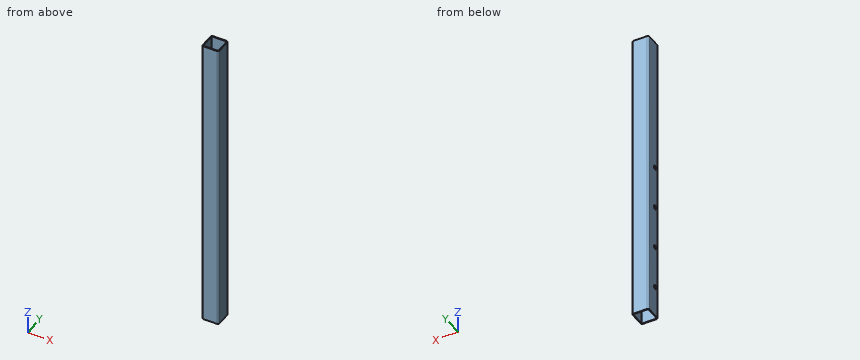
Autodesk Inventor part; units mm, degrees
ref_plane "Piano iniziale" through (0, 0, 0) normal (0, 0, 1) x (1, 0, 0)
ref_plane "Piano finale" through (0, 0, 720) normal (0, 0, 1) x (1, 0, 0)
ref_plane "YZ Plane" through (0, 0, 0) normal (1, 0, 0) x (0, 1, 0)
ref_plane "Piano iniziale" through (0, 0, 0) normal (0, 0, 1) x (1, 0, 0)
ref_plane "Piano finale" through (0, 0, 720) normal (0, 0, 1) x (1, 0, 0)
sketch "Schizzo" plane through (0, 0, 0) normal (0, 0, 1) x (1, 0, 0)
  line L0 (-20, -16) -> (-20, 16)
  line L1 (-16, 20) -> (16, 20)
  line L2 (20, 16) -> (20, -16)
  line L3 (16, -20) -> (-16, -20)
  arc A0 (-20, -16) -> (-16, -20) centre (-16, -16) ccw
  arc A1 (20, 16) -> (16, 20) centre (16, 16) ccw
  arc A2 (-16, 20) -> (-20, 16) centre (-16, 16) ccw
  arc A3 (16, -20) -> (20, -16) centre (16, -16) ccw
  arc A4 (-16, 18) -> (-18, 16) centre (-16, 16) ccw
  line L4 (-16, 18) -> (16, 18)
  arc A5 (18, 16) -> (16, 18) centre (16, 16) ccw
  line L5 (18, 16) -> (18, -16)
  arc A6 (16, -18) -> (18, -16) centre (16, -16) ccw
  line L6 (16, -18) -> (-16, -18)
  arc A7 (-18, -16) -> (-16, -18) centre (-16, -16) ccw
  line L7 (-18, -16) -> (-18, 16)
  line L8 (0, 29.1598) -> (0, -29.1598) construction
  line L9 (-29.1598, 0) -> (29.1598, 0) construction
  dimension "d7" = 4
  dimension "d9" = 40
  dimension "d11" = 40
  dimension "d12" = 2
  dimension "d15" = 20
  dimension "d16" = 20
extrude "Corpo" add sketch "Schizzo" along normal up to surface (720 mm away) from surface at 0
sketch "Sketch3" plane through (0, 0, 0) normal (0, 0, 1) x (1, 0, 0)
  line L0 (0, 0) -> (10, 0)
ref_plane "Work Plane3" through (0, 0, 0) normal (0, -1, 0) x (1, 0, 0)
sketch "Sketch4" plane through (0, 0, 0) normal (0, -1, 0) x (1, 0, 0)
  line L0 (-2, 0) -> (12, 0)
  line L1 (-2, 720) -> (12, 720)
  dimension "d18" = 720
sketch "Schizzo5" plane through (-20, 16, 0) normal (-1, 0, 0) x (0, 0, 1)
  line L0 (0, -36) -> (720, -36)
  line L1 (0, -32) -> (0, 0)
  point P0 (0, -16)
  point P1 (75, -23.5)
  point P2 (285, -23.5)
  point P3 (390, -23.5)
  point P4 (180, -23.5)
  dimension "d22" = 105
  dimension "d30" = 12.5
  dimension "d31" = 75
  dimension "d32" = 105
  dimension "d33" = 105
hole "Foro1" at (-20, -7.5, 75) at (-20, -7.5, 285) at (-20, -7.5, 390) at (-20, -7.5, 180) direction (1, 0, 0) diameter 10 depth 5 tip angle 118
equation "\"d7\" = G_IR"
equation "\"d9\" = G_W"
equation "\"d11\" = G_H"
equation "\"d12\" = G_T"
equation "\"d15\" = 0.5 * d9"
equation "\"d16\" = 0.5 * d11"
equation "\"d3\" = G_L"
equation "\"G_W\" = 40"
equation "\"G_H\" = 40"
equation "\"G_T\" = 2"
equation "\"G_IR\" = 4"
equation "\"G_L\" = d18"
equation "\"G_OFFSET_START\" = 0"
equation "\"G_OFFSET_END\" = 0"
properties part number "ISO 10799-2 - 40x40x2 - 720" material "Acciaio, Dolce"
Can you work these out from the model? Positions are in its coordinate system, mm. Give positions to 0.01 mm unless a question says otherwise; leave off trailing zeros. Order: outer loops, then holes, each group sorted by start corner. A loop starts at its lowest first (then second) coordinate and runs counter-clockwise, first axis right, second up. Notation, with made-up numbers: (-27, 88) - (-12, 88) arc R21 ccw to (-12, 114) - close; hole circle Ø10 at (53.5, -7.5). An arc over 180 degrees is marked (long way). Use a Markdown table: item, result. Add a question column.
Q1. Please list where these lines run through material, in increasing order: line 1 along Z through (x, y) = (-19.45, -7.5); line 2 along X through (y, z) = (-15, 607.5).
Q2. I'm going to push a flat-ended pin straight in: pin 1 (13 mm diameter, centred on y = -7.5, z = 180, fed in from -X). Where does the tip first touch, or does it pass through?
Q3. If we section it at A-A on y = 5: Write out the boundary of the cut face in (x, z).
Q4. If we section it at B-B on z = 100: Write out the boundary of the cut face in (x, y), plus the area to 3 significant figures.
Answers follow:
| question | item | result |
|---|---|---|
| 1 | line 1 | z = 0 to 70, 80 to 175, 185 to 280, 290 to 385, 395 to 720 |
| 1 | line 2 | x = -20 to -18, 18 to 20 |
| 2 | pin 1 | stops at x = -20 |
| 3 | outline | (-20, 0) - (-18, 0) - (-18, 720) - (-20, 720) - close; (18, 0) - (20, 0) - (20, 720) - (18, 720) - close |
| 4 | outline | (-20, -16) arc R4 ccw to (-16, -20) - (16, -20) arc R4 ccw to (20, -16) - (20, 16) arc R4 ccw to (16, 20) - (-16, 20) arc R4 ccw to (-20, 16) - close; hole (-18, -16) arc R2 ccw to (-16, -18) - (16, -18) arc R2 ccw to (18, -16) - (18, 16) arc R2 ccw to (16, 18) - (-16, 18) arc R2 ccw to (-18, 16) - close |
| 4 | area | 294 mm^2 |
